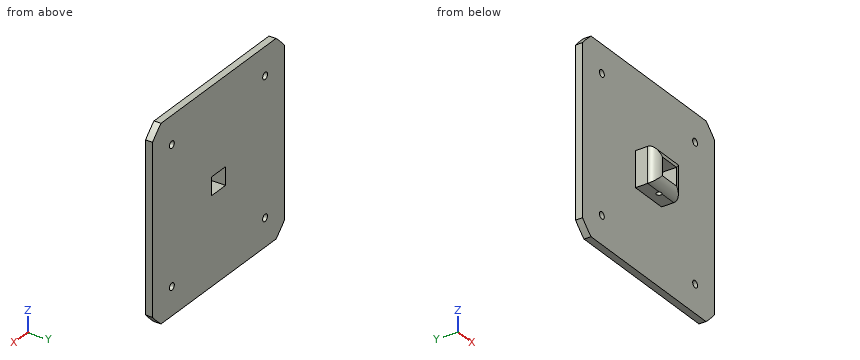
```python
from build123d import *

# Parameters (mm, degrees)
BOSS_EXTRUDE1_DEPTH       = 4
F_4_0MM_DOWEL_HOLE2_D     = 4
SKETCH7_W                 = 11.8
SKETCH7_H                 = 10.3
CUT_EXTRUDE1_DEPTH        = 10
SKETCH8_W                 = 21.8
SKETCH8_H                 = 20.3
SKETCH8_W_2               = 11.8
SKETCH8_H_2               = 10.3
BOSS_EXTRUDE2_DEPTH       = 12
FILLET1_START             = -10.15
FILLET1_DEPTH             = 20.3
FILLET1_START_2           = -12
FILLET1_2_DEPTH           = 24
F_3_0MM_DOWEL_HOLE1_D     = 3
F_3_0MM_DOWEL_HOLE1_DEPTH = 5


with BuildPart() as part:
    # Sketch1 → Boss-Extrude1 (new body)
    with BuildSketch(Plane(origin=(0, 0, 0), x_dir=(1, 0, 0), z_dir=(0, 1, 0))):
        with BuildLine():
            Line((55, 48), (55, -48))
            ThreePointArc((55, -48), (51.618795027, -51.618795027), (48, -55))
            Line((48, -55), (-48, -55))
            ThreePointArc((-48, -55), (-51.618795027, -51.618795027), (-55, -48))
            Line((-55, -48), (-55, 48))
            ThreePointArc((-55, 48), (-51.618795027, 51.618795027), (-48, 55))
            Line((-48, 55), (48, 55))
            ThreePointArc((48, 55), (51.618795027, 51.618795027), (55, 48))
        make_face()
    extrude(amount=BOSS_EXTRUDE1_DEPTH)

    # Ø4.0mm Dowel Hole2 (through all)
    with Locations(Plane(origin=(0, 4, 0), x_dir=(1, 0, 0), z_dir=(0, 1, 0))):
        with Locations((38.890872965, 38.890872965), (38.890872965, -38.890872965), (-38.890872965, -38.890872965), (-38.890872965, 38.890872965)):
            Hole(F_4_0MM_DOWEL_HOLE2_D / 2)

    # Sketch7 → Cut-Extrude1 (cut)
    with BuildSketch(Plane.XZ):
        Rectangle(SKETCH7_W, SKETCH7_H)
    extrude(amount=-CUT_EXTRUDE1_DEPTH, mode=Mode.SUBTRACT)

    # Sketch8 → Boss-Extrude2 (add)
    with BuildSketch(Plane.XZ):
        Rectangle(SKETCH8_W, SKETCH8_H)
        Rectangle(SKETCH8_W_2, SKETCH8_H_2, mode=Mode.SUBTRACT)
    extrude(amount=BOSS_EXTRUDE2_DEPTH)

    # Fillet1: read off the stored shape, not the designer's step
    # Fillet1 outline → Fillet1 (cut)
    with BuildSketch(Plane.XY.offset(FILLET1_START)):
        with BuildLine():
            Line((10.9, -12), (10.9, -7))
            ThreePointArc((10.9, -7), (9.435533906, -10.535533906), (5.9, -12))
            Line((5.9, -12), (10.9, -12))
        make_face()
        with BuildLine():
            Line((-10.9, -12), (-5.9, -12))
            ThreePointArc((-5.9, -12), (-9.435533906, -10.535533906), (-10.9, -7))
            Line((-10.9, -7), (-10.9, -12))
        make_face()
    extrude(amount=FILLET1_DEPTH, mode=Mode.SUBTRACT)

    # Fillet1 2 outline → Fillet1 2 (cut)
    with BuildSketch(Plane.YZ.offset(FILLET1_START_2)):
        with BuildLine():
            ThreePointArc((-12, 5.15), (-10.535533906, 8.685533906), (-7, 10.15))
            Line((-7, 10.15), (-12, 10.15))
            Line((-12, 10.15), (-12, 5.15))
        make_face()
        with BuildLine():
            Line((-12, -10.15), (-7, -10.15))
            ThreePointArc((-7, -10.15), (-10.535533906, -8.685533906), (-12, -5.15))
            Line((-12, -5.15), (-12, -10.15))
        make_face()
    extrude(amount=FILLET1_2_DEPTH, mode=Mode.SUBTRACT)

    # Ø3.0mm Dowel Hole1
    with Locations(Plane(origin=(0, 0, -10.15), x_dir=(-1, 0, 0), z_dir=(0, 0, -1))):
        with Locations((0, -6)):
            Hole(F_3_0MM_DOWEL_HOLE1_D / 2, depth=F_3_0MM_DOWEL_HOLE1_DEPTH)


solid = part.part
```
Input: part model. Units: mm. Frame: model coordinates. Coordinates: 2 decimals unless noted, no trailing zeros. Loops run counter-clockwise (first coordinate to the right, second up) from the corner with the lowest first, then second, coordinate; pieces in that order, holes last.
Q1. Line query: line 1 along Z through (x, y) = (-4.5, 3); line 2 along Z through (x, y) = (-2, -3); line 3 along X through (y, z) = (-6, -8.95). Output: solid intervals per line, ascending.
Results are:
line 1: z = -55 to -5.15, 5.15 to 55
line 2: z = -10.15 to -5.15, 5.15 to 10.15
line 3: x = -10.9 to -1.5, 1.5 to 10.9
Q2. Contact query for flat-ended pins moving along their axis: pin 1 (6 mm diameter, centred on y = -4.5, z = -9, fed in from +X); pin 2 (3.5 mm diameter, centred on x = -2, y = -6, fed in from +Z); pin 3 (5.5 mm diameter, centred on y = -4.5, z = -4.5, fed in from -X). Output: stop coordinate, or through.
Results are:
pin 1: stops at x = 10.9
pin 2: stops at z = 10.15
pin 3: stops at x = -10.9
Q3. Section C-C, the plane z = 23. Return the cut outline in (x, y), and give its area (3 significant figures).
Results are:
outline: (-55, 0) - (55, 0) - (55, 4) - (-55, 4) - close
area: 440 mm2
Q4. Section A-A, the plane z = 7. Return the cut outline in (x, y).
Results are:
outline: (-55, 0) - (-10.9, 0) - (-10.9, -7) arc R5 ccw to (-7.75, -11.65) - (7.75, -11.65) arc R5 ccw to (10.9, -7) - (10.9, 0) - (55, 0) - (55, 4) - (-55, 4) - close
Q5. Section B-B, the plane x = -18. Return the cut outline in (y, z).
Results are:
outline: (0, -55) - (4, -55) - (4, 55) - (0, 55) - close
